```python
from build123d import *


with BuildPart() as part:
    # Sketch1 → Revolve1 (revolve)
    with BuildSketch(Plane(origin=(0, 0, 0), x_dir=(0, 0, -1), z_dir=(1, 0, 0)), mode=Mode.PRIVATE) as revolve1_sk:
        with BuildLine():
            Line((-1.5, 3), (-2, 3))
            Line((-2, 3), (-2, 2))
            Line((-2, 2), (2, 2))
            Line((2, 2), (2, 3))
            Line((2, 3), (1.5, 3))
            Line((1.5, 3), (1.5, 14.545643943))
            ThreePointArc((1.5, 14.545643943), (1.658374588, 15.085705668), (2.083333333, 15.454703286))
            ThreePointArc((2.083333333, 15.454703286), (0, 25), (-2.083333333, 15.454703286))
            ThreePointArc((-2.083333333, 15.454703286), (-1.658374588, 15.085705668), (-1.5, 14.545643943))
            Line((-1.5, 14.545643943), (-1.5, 3))
        make_face()
    revolve(revolve1_sk.sketch.rotate(Axis((0, 0, -18.162203791), (0, 0, 1)), 90), axis=Axis((0, 0, -18.162203791), (0, 0, 1)))  # turned: the seam where the file's is


solid = part.part
```
Work out the finished part from the listing and answer in its coordinate system (mm). A direction names the side the tool comes from. Coordinates: 2 decimals unless noted, no trailing zeros. Write each loop counter-clockwise with the first axis right and the second up, starting at its lowest first coordinate (ties: lowest second). Pieces come first, ordered by that corner, then holes.
Q1. A cutting plane is placed at C-C, the plane z = -4. Give the vertices of the cut face in (x, y), then the cut area to 3 significant figures.
Q2. Each of these flat-tipped pins is pushed along its axis until it touches: pin 1 Ø3 at (x, z) = (17.5, 4) entering from -Y; pin 2 Ø3 at (y, z) = (-5.5, 3.5) entering from -X; pin 3 Ø8.5 at (x, y) = (-3.5, -3.5) entering from +Z; pin 4 Ø1.8 at (x, y) = (-0.5, 0) entering from -Z. Where does it stop, or does it pass through?
Q3. A cutting plane is placed at A-A, the plane y = 0. Give the vertices of the cut face in (x, z), then the cut area to 3 significant figures.
Q4. A cutting plane is placed at D-D, the plane z = 3.25. Give the vertices of the cut face in (x, y), then the cut area to 3 significant figures.
Q5. Determine the mould class of faces 1 (the face through (-0.2, -3.4, -1.5)), 2 (the face through (-2.86, -0.9, -1.75)) for opening direction Y: released by +Y, released by -Y, zero draft, split by the parting line, or undercut.
Q6. Which of the six approach directions +Z, -Z, +X, -X, +Y, -Y give full straight-line access (tool end or side, diameter ignored) to faces 3 (the face through (0.2, -3.4, 1.5)), 4 (the face through (1, 2, -2)), 5 (the face through (0, 2, 0))?
Q7. Find the intervals of material crossed by line 1 (Y direction, x = 0, z = -0.3); line 2 (Y direction, x = -19.5, z = -2.5); line 3 (Y direction, x = 6.5, z = -3.25), in increasing order.
Findings below:
1. outline: circle Ø46 at (0, 0); hole circle Ø34 at (0, 0)
1. area: 754 mm2
2. pin 1: stops at y = -17.55
2. pin 2: stops at x = -24.03
2. pin 3: stops at z = 2
2. pin 4: passes through
3. outline: (-15.45, -2.08) arc R1 cw to (-14.55, -1.5) - (-3, -1.5) - (-3, -2) - (-2, -2) - (-2, 2) - (-3, 2) - (-3, 1.5) - (-14.55, 1.5) arc R1 cw to (-15.45, 2.08) arc R5 ccw (long way) to start; (2, -2) - (3, -2) - (3, -1.5) - (14.55, -1.5) arc R1 cw to (15.45, -2.08) arc R5 ccw (long way) to (15.45, 2.08) arc R1 cw to (14.55, 1.5) - (3, 1.5) - (3, 2) - (2, 2) - close
3. area: 238 mm2
4. outline: circle Ø47.6 at (0, 0); hole circle Ø32.4 at (0, 0)
4. area: 955 mm2
5. face 1: undercut
5. face 2: undercut
6. face 3: +Z
6. face 4: -Z
6. face 5: +Z, -Z
7. line 1: y = -24.99 to -2, 2 to 24.99
7. line 2: y = -14.55 to 14.55
7. line 3: y = -22.89 to -14.84, 14.84 to 22.89
